Input: part model. Units: mm. Frame: model coordinates. A direction names the side the tool comes from. Give positions to 0.01 mm unless a question says otherwise; leave off trailing zeros. Loops run counter-clockwise (first coordinate to the right, second up) from the corner with the lowest first, then second, coordinate; pieces in that order, holes last. Notation, with made-up numbers: M -28,71 L 1,71 A13 ccw 1,96 Z; hole C 0,74.25 d9. An arc over 180 degrees is marked long. Answer as a JSON object with one key per item and string values. Group by question number.
1) Access query for faces 1 (the flat face through (3, 13, -23)), 2 (the flat face through (3, 9, -5)), 3 (the flat face through (3, 42, -23)), 4 (the flat face through (3, 18, -23)), 5 (the flat face through (0, 20, -12)). Directions: +Z, -Z, +X, -X, +Y, -Y. A direction counts if a zero-diameter tool reaches every point of the face in a straight line with its end or side. Return the directions, or none.
2) Section query C-C on z = -3. Return loops of the section in (x, y).
3) Section query A-A on z = -23. Return loops of the section in (x, y).
4) Ray query, L1, parallel to Y at x = 1.55, z = -21.5; L2, parallel to Y at x = 1.5, z = -2.75; L3, parallel to Y at x = 3.15, z = -17. Return the intervals inside material, ascending.
5) Draft query along Z for faces 6 (the cylindrical face through (3, 18, -20)), 7 (the flat face through (3, 3.3, -10)), 8 (the flat face through (2, 28, -20)). Return one class per face: +Z half, -Z half, draft (parallel to the pull), parting line (faces both ways), or undercut.
6) Section query D-D on y = 16. Return loops of the section in (x, z).
7) First-contact query: P1, Ø0.8, axis at x = 2, y = 44, coming from the -Z side; P2, Ø1.1, axis at x = 2.5, z = -1.5, coming from the +Y side; P3, Ø2, axis at x = 4, z = -5.5, coming from the +Y side. Flat tips, straight axial feed; report the tip coordinate or a pass-through.
8) Section query B-B on x = 2.65. Return loops of the section in (y, z).
from build123d import *

# Parameters (mm, degrees)
EXTRUDE_1_DEPTH     = 5
SKETCH_7_W          = 5
SKETCH_7_H          = 10.8
CUT_EXTRUDE_1_DEPTH = 5
SKETCH_8_W          = 15
SKETCH_8_H          = 3.3
CUT_EXTRUDE_2_DEPTH = 5
SKETCH_10_W         = 5
SKETCH_10_H         = 3.6
EXTRUDE_2_DEPTH     = 5
SKETCH_9_R          = 1
CUT_EXTRUDE_3_DEPTH = 5
SKETCH_15_W         = 5
SKETCH_15_H         = 4
SKETCH_15_H_2       = 5
EXTRUDE_6_DEPTH     = 5
SKETCH_11_W         = 5
SKETCH_11_H         = 5
SKETCH_11_H_2       = 4
EXTRUDE_3_DEPTH     = 5
SKETCH_12_R         = 1
CUT_EXTRUDE_4_DEPTH = 5
FILLET_1_R          = 0.5


with BuildPart() as part:
    # 스케치1 → 보스-돌출1 (new body)
    with BuildSketch(Plane(origin=(0, 0, 0), x_dir=(0, 0, -1), z_dir=(1, 0, 0))):
        Polygon((0, 0), (0, 12), (17, 45), (20, 45), (20, 0), align=None)
    extrude(amount=EXTRUDE_1_DEPTH)

    # 스케치7 → 컷-돌출1 (cut)
    with BuildSketch(Plane(origin=(5, 0, 0), x_dir=(0, 0, -1), z_dir=(1, 0, 0))):
        with Locations((2.5, 5.4)):
            Rectangle(SKETCH_7_W, SKETCH_7_H)
    extrude(amount=-CUT_EXTRUDE_1_DEPTH, mode=Mode.SUBTRACT)

    # 스케치8 → 컷-돌출2 (cut)
    with BuildSketch(Plane(origin=(5, 0, 0), x_dir=(0, 0, -1), z_dir=(1, 0, 0))):
        with Locations((12.5, 1.65)):
            Rectangle(SKETCH_8_W, SKETCH_8_H)
    extrude(amount=-CUT_EXTRUDE_2_DEPTH, mode=Mode.SUBTRACT)

    # 스케치10 → 보스-돌출2 (add)
    with BuildSketch(Plane(origin=(5, 0, 0), x_dir=(0, 0, -1), z_dir=(1, 0, 0))):
        with Locations((2.5, 5.1)):
            Rectangle(SKETCH_10_W, SKETCH_10_H)
    extrude(amount=-EXTRUDE_2_DEPTH)

    # 스케치9 → 컷-돌출3 (cut)
    with BuildSketch(Plane(origin=(5, 0, 0), x_dir=(0, 0, -1), z_dir=(1, 0, 0))):
        with Locations((4.292893219, 10.092893219)):
            Circle(SKETCH_9_R)
        with Locations((4.292893219, 7.607106781)):
            Circle(SKETCH_9_R)
    extrude(amount=-CUT_EXTRUDE_3_DEPTH, mode=Mode.SUBTRACT)

    # 스케치15 → 보스-돌출6 (add)
    with BuildSketch(Plane(origin=(5, 0, 0), x_dir=(0, 0, -1), z_dir=(1, 0, 0))):
        with Locations((22.5, 40)):
            Rectangle(SKETCH_15_W, SKETCH_15_H)
        with Locations((22.5, 15.5)):
            Rectangle(SKETCH_15_W, SKETCH_15_H_2)
    extrude(amount=-EXTRUDE_6_DEPTH)

    # 스케치11 → 보스-돌출3 (add)
    with BuildSketch(Plane(origin=(5, 0, 0), x_dir=(0, 0, -1), z_dir=(1, 0, 0))):
        with Locations((22.5, 15.5)):
            Rectangle(SKETCH_11_W, SKETCH_11_H)
        with Locations((22.5, 40)):
            Rectangle(SKETCH_11_W, SKETCH_11_H_2)
    extrude(amount=-EXTRUDE_3_DEPTH)

    # 스케치12 → 컷-돌출4 (cut)
    with BuildSketch(Plane(origin=(5, 0, 0), x_dir=(0, 0, -1), z_dir=(1, 0, 0))):
        with Locations((20.707106781, 18.707106781)):
            Circle(SKETCH_12_R)
        with Locations((20.707106781, 12.292893219)):
            Circle(SKETCH_12_R)
        with Locations((20.707106781, 37.292893219)):
            Circle(SKETCH_12_R)
        with Locations((20.707106781, 42.707106781)):
            Circle(SKETCH_12_R)
    extrude(amount=-CUT_EXTRUDE_4_DEPTH, mode=Mode.SUBTRACT)

    # 필렛1
    fillet_1_edges = [part.edges().sort_by_distance(p)[0] for p in [
        (2.5, 13, -25),
        (2.5, 38, -25),
        (2.5, 18, -25),
        (2.5, 42, -25),
        (2.5, 45, -17),
    ]]
    fillet(fillet_1_edges, radius=FILLET_1_R)


solid = part.part
Output:
{
 "1": {"face 1": "-Z, +X, -X, -Y", "face 2": "+Z, +X, -X", "face 3": "-Z, +X, -X, +Y", "face 4": "-Z, +X, -X", "face 5": "+Z, -Z, -X, +Y, -Y"},
 "2": {"outline": "M 0,3.3 L 5,3.3 L 5,6.9 L 0,6.9 Z; M 0,10.8 L 5,10.8 L 5,17.82 L 0,17.82 Z"},
 "3": {"outline": "M 0,13 L 5,13 L 5,18 L 0,18 Z; M 0,38 L 5,38 L 5,42 L 0,42 Z"},
 "4": {"L1": "y = 13 to 18, 38 to 42", "L2": "y = 3.3 to 6.9, 10.8 to 17.34", "L3": "y = 3.3 to 44.9"},
 "5": {"face 6": "undercut", "face 7": "draft", "face 8": "-Z half"},
 "6": {"outline": "M 0,-25 L 5,-25 L 5,-2.06 L 0,-2.06 Z"},
 "7": {"P1": "stops at z = -20", "P2": "stops at y = 15.98", "P3": "stops at y = 24.62"},
 "8": {"outline": "M 3.3,-20 L 11.59,-20 A1 cw 13,-21.41 L 13,-24.5 A0.5 ccw 13.5,-25 L 17.5,-25 A0.5 ccw 18,-24.5 L 18,-21.41 A1 cw 19.41,-20 L 36.59,-20 A1 cw 38,-21.41 L 38,-24.5 A0.5 ccw 38.5,-25 L 41.5,-25 A0.5 ccw 42,-24.5 L 42,-21.41 A1 cw 43.41,-20 L 45,-20 L 45,-17.3 A0.5 ccw 44.73,-16.86 L 12,0 L 10.8,0 L 10.8,-3.59 A1 cw 9.39,-5 L 8.31,-5 A1 cw 6.9,-3.59 L 6.9,0 L 3.3,0 Z"}
}
